```python
from build123d import *

# Parameters (mm, degrees)
SKETCH_1_W          = 500.8
SKETCH_1_H          = 300.8
EXTRUDE_1_DEPTH     = 4.75
SKETCH_2_W          = 25.4
SKETCH_2_H          = 25.4
SKETCH_2_W_2        = 4.75
SKETCH_2_H_2        = 80
SKETCH_2_W_3        = 5.096596069
CUT_EXTRUDE_1_DEPTH = 10


with BuildPart() as part:
    # 草圖1 → 填料-伸長1 (new body)
    with BuildSketch(Plane.XY):
        Rectangle(SKETCH_1_W, SKETCH_1_H)
    extrude(amount=EXTRUDE_1_DEPTH)

    # 草圖2 → 除料-伸長1 (cut)
    with BuildSketch(Plane(origin=(0, 0, 0), x_dir=(-1, 0, 0), z_dir=(0, 0, -1))):
        with Locations((-237.7, 137.7)):
            Rectangle(SKETCH_2_W, SKETCH_2_H)
        with Locations((-237.7, -137.7)):
            Rectangle(SKETCH_2_W, SKETCH_2_H)
        with Locations((237.7, 137.7)):
            Rectangle(SKETCH_2_W, SKETCH_2_H)
        with Locations((237.7, -137.7)):
            Rectangle(SKETCH_2_W, SKETCH_2_H)
        with Locations((-222.625, 65.4)):
            Rectangle(SKETCH_2_W_2, SKETCH_2_H_2)
        with Locations((-222.625, -65.4)):
            Rectangle(SKETCH_2_W_2, SKETCH_2_H_2)
        with Locations((222.625, 65.4)):
            Rectangle(SKETCH_2_W_2, SKETCH_2_H_2)
        with Locations((222.625, -64.4)):
            Rectangle(SKETCH_2_W_2, SKETCH_2_H_2)
        with Locations((187.875, 65.4)):
            Rectangle(SKETCH_2_W_2, SKETCH_2_H_2)
        with Locations((187.875, -64.4)):
            Rectangle(SKETCH_2_W_2, SKETCH_2_H_2)
        with Locations((-109.565361966, 65.4)):
            Rectangle(SKETCH_2_W_3, SKETCH_2_H_2)
        with Locations((-74.468765897, 65.4)):
            Rectangle(SKETCH_2_W_3, SKETCH_2_H_2)
        with Locations((40.781234104, 65.4)):
            Rectangle(SKETCH_2_W_3, SKETCH_2_H_2)
        with Locations((70.434638035, 65.4)):
            Rectangle(SKETCH_2_W_3, SKETCH_2_H_2)
    extrude(amount=-CUT_EXTRUDE_1_DEPTH, mode=Mode.SUBTRACT)


solid = part.part
```
For this review, take the finished solid that the model builds, in its own axes (mm). Round coordinates to 2 decimals unless told otherwise and drop trailing zeros. Write each loop counter-clockwise with the first axis right and the second up, starting at its lowest first coordinate (ties: lowest second). Pieces come first, ordered by that corner, then holes. Notation, with made-up numbers: (14.5, 86.25) - (35.5, 86.25) arc R30 ccw to (35.5, 121.25) - close; hole circle Ø7 at (-38, 65). An arc over 180 degrees is marked (long way). Answer as a JSON object with one key per item and string values.
1. For pin 1 Ø2.5 at (y, z) = (-134.5, 3.5) entering from -X, flat-tipped, find the tip position at first contact; note if it passes through.
Response values:
{"pin 1": "stops at x = -225"}
2. To check wall thickness, follow line 1 along X through (y, z) = (-90, 0.8); line 2 along X through (y, z) = (-134, 1.7). State the ranges of each line that lie inside material, in increasing order.
Response values:
{"line 1": "x = -250.4 to -225, -220.25 to -190.25, -185.5 to 220.25, 225 to 250.4", "line 2": "x = -225 to 225"}
3. We need section A-A on y = 100.5. Count the separate pieces of the cut face and the enclosed holes in it, then the cut area to 3 significant figures.
Response values:
{"separate pieces": "8", "enclosed holes": "0", "area": "2,210 mm2"}
4. We need section B-B on y = -57. Give the boundary of the cut face in (x, z).
Response values:
{"outline": "(-250.4, 0) - (-225, 0) - (-225, 4.75) - (-250.4, 4.75) - close; (-220.25, 0) - (-190.25, 0) - (-190.25, 4.75) - (-220.25, 4.75) - close; (-185.5, 0) - (220.25, 0) - (220.25, 4.75) - (-185.5, 4.75) - close; (225, 0) - (250.4, 0) - (250.4, 4.75) - (225, 4.75) - close"}
